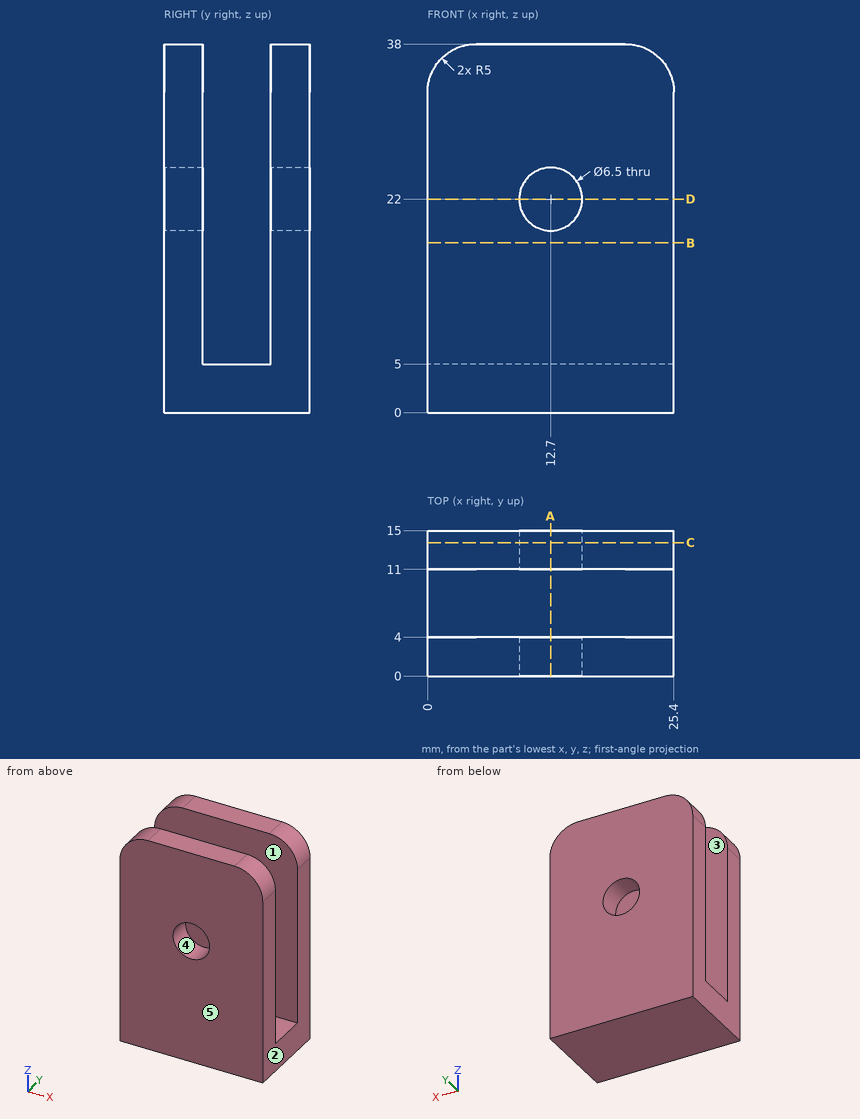
Print and shaded views of the part. All mm, measured from the part's lowest x, y and z. A direction names the side the tool comes from. Round coordinates to 2 decimals unless told otherwise and drop trailing zeros. Write each loop counter-clockwise with the first axis right and the second up, starting at its lowest first coordinate (ties: lowest second). Pieces come first, ordered by that corner, then holes. Notation, with made-up numbers: (79.5, -31.75) - (91.5, -31.75) arc R11 cw to (91.5, -12.75) - close; hole circle Ø6 at (-21.5, -6). An arc over 180 degrees is marked (long way). Write each question's results on one line, items separated by ' | '. Start each with the question number.
Item 1: Which spindle directions (+Z, -Z, +X, -X, +Y, -Y) get a long thin tool onto all of the face, cutting with end or side? Do the marked faces 1 and 2. Say none if no direction does.
Item 2: Wall check: L1, parallel to Y at x = 15, z = 13.5; L2, parallel to Z at x = 12.7, y = 12.15; L3, parallel to Z at x = 7.5, y = 4.25. Give the ranges that are in metal, low to high. Write a range as [from, to].
Item 3: Saw through at A-A (x = 12.7). Write the cut outline in (y, z).
Item 4: Saw through at D-D (z = 22). Write the cut outline in (x, y), and give its area (3 significant figures).
Item 5: Saw through at C-C (y = 13.75). Write the cut outline in (x, z), and give its area (3 significant figures).
Item 6: Saw through at B-B (z = 17.5). Write the cut outline in (x, y), and give its area (3 significant figures).
Item 7: Drop flat-ended pins along their axis: P1, Ø4, axis at x = 12.7, z = 22, coming from the +Y side; P2, Ø2, axis at x = 17.5, y = 8, coming from the +Z side. Give the stop position or say it passes through.
Item 8: Mould opens along Y. For the marked faces 3, 4 and 5 say: pulls with the +Y half, pulls with the -Y half, needs draft (parallel to the pull), parting line crosses it, or undercut.
Results are:
1) face 1: +Z, +X, -X | face 2: +Z, -Z, +X, +Y, -Y
2) L1: y = [0, 4], [11, 15] | L2: z = [0, 18.75], [25.25, 38] | L3: z = [0, 5]
3) outline: (0, 0) - (15, 0) - (15, 18.75) - (11, 18.75) - (11, 5) - (4, 5) - (4, 18.75) - (0, 18.75) - close; (0, 25.25) - (4, 25.25) - (4, 38) - (0, 38) - close; (11, 25.25) - (15, 25.25) - (15, 38) - (11, 38) - close
4) outline: (0, 0) - (9.45, 0) - (9.45, 4) - (0, 4) - close; (0, 11) - (9.45, 11) - (9.45, 15) - (0, 15) - close; (15.95, 0) - (25.4, 0) - (25.4, 4) - (15.95, 4) - close; (15.95, 11) - (25.4, 11) - (25.4, 15) - (15.95, 15) - close | area: 151 mm²
5) outline: (0, 0) - (25.4, 0) - (25.4, 33) arc R5 ccw to (20.4, 38) - (5, 38) arc R5 ccw to (0, 33) - close; hole circle Ø6.5 at (12.7, 22) | area: 921 mm²
6) outline: (0, 0) - (25.4, 0) - (25.4, 4) - (0, 4) - close; (0, 11) - (25.4, 11) - (25.4, 15) - (0, 15) - close | area: 203 mm²
7) P1: passes through | P2: stops at z = 5
8) face 3: undercut | face 4: needs draft | face 5: pulls with the -Y half
